Geometry check sheet. Reference: the model listing, model coordinates, mm. A direction names the side the tool comes from. Coordinates: 2 decimals unless noted, no trailing zeros. Loops run counter-clockwise (first coordinate to the right, second up) from the corner with the lowest first, then second, coordinate; pieces in that order, holes last. Notation, with made-up numbers: (-37, 65.5) -> (16, 65.5) arc R14 cw to (16, 87.5) -> close; hole circle Ø8 at (-17, 50). An arc over 180 degrees is marked (long way). Answer as a JSON object with one key per item and string values.
Autodesk Inventor part; units mm, degrees
ref_plane "YZ Plane" through (0, 0, 0) normal (1, 0, 0) x (0, 1, 0)
ref_plane "XZ Plane" through (0, 0, 0) normal (0, 1, 0) x (-1, 0, 0)
ref_plane "XY Plane" through (0, 0, 0) normal (0, 0, 1) x (1, 0, 0)
sketch "Sketch1" plane through (0, 0, 0) normal (0, 1, 0) x (-1, 0, 0)
  line L0 (-25.25, 42.75) -> (25.25, 42.75)
  line L1 (28.25, 39.75) -> (28.25, -40.75)
  line L2 (26.25, -42.75) -> (-25.25, -42.75)
  line L3 (-28.25, -39.75) -> (-28.25, 39.75)
  line L4 (-28.25, 42.75) -> (28.25, -42.75) construction
  line L5 (28.25, 42.75) -> (-28.25, -42.75) construction
  arc A0 (26.25, -42.75) -> (28.25, -40.75) centre (26.25, -40.75) ccw
  arc A1 (-28.25, -39.75) -> (-25.25, -42.75) centre (-25.25, -39.75) ccw
  arc A2 (-25.25, 42.75) -> (-28.25, 39.75) centre (-25.25, 39.75) ccw
  arc A3 (28.25, 39.75) -> (25.25, 42.75) centre (25.25, 39.75) ccw
  line L6 (30.25, -40.75) -> (30.25, 39.75)
  arc A4 (30.25, 39.75) -> (25.25, 44.75) centre (25.25, 39.75) ccw
  line L7 (25.25, 44.75) -> (-25.25, 44.75)
  arc A5 (-25.25, 44.75) -> (-30.25, 39.75) centre (-25.25, 39.75) ccw
  line L8 (-30.25, 39.75) -> (-30.25, -39.75)
  arc A6 (-30.25, -39.75) -> (-25.25, -44.75) centre (-25.25, -39.75) ccw
  line L9 (-25.25, -44.75) -> (26.25, -44.75)
  arc A7 (26.25, -44.75) -> (30.25, -40.75) centre (26.25, -40.75) ccw
  point P0 (0, 0)
  dimension "d0" = 56.5
  dimension "d1" = 85.5
  dimension "d2" = 2
  dimension "d3" = 3
  dimension "d4" = 2
extrude "Extrusion1" add sketch "Sketch1" along normal blind 3
sketch "Sketch2" plane through (0, 0, 0) normal (0, -1, 0) x (1, 0, 0)
  arc A0 (-25.25, 44.75) -> (-30.25, 39.75) centre (-25.25, 39.75) ccw
  line L0 (-25.25, 44.75) -> (25.25, 44.75)
  arc A1 (30.25, 39.75) -> (25.25, 44.75) centre (25.25, 39.75) ccw
  line L1 (30.25, 39.75) -> (30.25, -39.75)
  arc A2 (25.25, -44.75) -> (30.25, -39.75) centre (25.25, -39.75) ccw
  line L2 (25.25, -44.75) -> (-26.25, -44.75)
  arc A3 (-30.25, -40.75) -> (-26.25, -44.75) centre (-26.25, -40.75) ccw
  line L3 (-30.25, -40.75) -> (-30.25, 39.75)
  line L4 (-26.25, -44.75) -> (25.25, -44.75)
  line L5 (30.25, -39.75) -> (30.25, 39.75)
  line L6 (25.25, 44.75) -> (-25.25, 44.75)
  line L7 (-30.25, 39.75) -> (-30.25, -40.75)
  line L8 (-30, -44.5) -> (30, 44.5) construction
  line L9 (30, -44.5) -> (-30, 44.5) construction
  arc A4 (-25.25, 44.75) -> (-30.25, 39.75) centre (-25.25, 39.75) ccw
  arc A5 (30.25, 39.75) -> (25.25, 44.75) centre (25.25, 39.75) ccw
  arc A6 (25.25, -42.75) -> (28.25, -39.75) centre (25.25, -39.75) ccw
  arc A7 (25.25, -44.75) -> (30.25, -39.75) centre (25.25, -39.75) ccw
  arc A8 (-30.25, -40.75) -> (-26.25, -44.75) centre (-26.25, -40.75) ccw
  line L10 (25.25, 40.75) -> (-25.25, 40.75)
  arc A9 (-25.25, 40.75) -> (-26.25, 39.75) centre (-25.25, 39.75) ccw
  line L11 (-26.25, 39.75) -> (-26.25, -40.75)
  line L12 (-26.25, -40.75) -> (25.25, -40.75)
  arc A10 (25.25, -40.75) -> (26.25, -39.75) centre (25.25, -39.75) ccw
  line L13 (26.25, -39.75) -> (26.25, 39.75)
  arc A11 (26.25, 39.75) -> (25.25, 40.75) centre (25.25, 39.75) ccw
  point P0 (0, 0)
  point P1 (-26.25, -40.75)
  dimension "d12" = 4
extrude "Extrusion2" add sketch "Sketch2" along normal blind 2.5
sketch "Sketch3" plane through (25.25, 3, -44.75) normal (0, 0, -1) x (-1, 0, 0)
  line L0 (51.5, -5.5) -> (51.5, 0)
  line L1 (51.5, 0) -> (0, 0)
  line L2 (0, 0) -> (0, 1.5)
  line L3 (0, 1.5) -> (51.5, 1.5)
  line L4 (51.5, 1.5) -> (51.5, 0)
  point P0 (25.25, -3)
  dimension "d9" = 1.5
extrude "Extrusion3" add sketch "Sketch3" against normal blind 2
sketch "Sketch4" plane through (0, -2.5, 0) normal (0, -1, 0) x (1, 0, 0)
  line L0 (25.25, 44.75) -> (-25.25, 44.75)
  line L1 (-30.25, 39.75) -> (-30.25, -40.75)
  line L2 (-26.25, -44.75) -> (25.25, -44.75)
  line L3 (30.25, -39.75) -> (30.25, 39.75)
  line L4 (30, 44.5) -> (-30, -44.5) construction
  line L5 (-30, 44.5) -> (30, -44.5) construction
  line L6 (-26.25, -44.75) -> (25.25, -44.75)
  line L7 (-30.25, 39.75) -> (-30.25, -40.75)
  arc A0 (25.25, -44.75) -> (30.25, -39.75) centre (25.25, -39.75) ccw
  arc A1 (-30.25, -40.75) -> (-26.25, -44.75) centre (-26.25, -40.75) ccw
  arc A2 (-25.25, 44.75) -> (-30.25, 39.75) centre (-25.25, 39.75) ccw
  arc A3 (30.25, 39.75) -> (25.25, 44.75) centre (25.25, 39.75) ccw
  arc A4 (25.25, -44.75) -> (30.25, -39.75) centre (25.25, -39.75) ccw
  line L8 (25.25, -40.75) -> (-26.25, -40.75)
  arc A5 (-30.25, -40.75) -> (-26.25, -44.75) centre (-26.25, -40.75) ccw
  arc A6 (-25.25, 44.75) -> (-30.25, 39.75) centre (-25.25, 39.75) ccw
  arc A7 (30.25, 39.75) -> (25.25, 44.75) centre (25.25, 39.75) ccw
  line L9 (25.25, 44.75) -> (-25.25, 44.75)
  point P0 (0, 0)
  point P1 (-30.25, 39.75)
  point P2 (-30.25, -40.75)
  point P3 (25.25, -44.75)
extrude "Extrusion4" add sketch "Sketch4" along normal blind 2.5
sketch "Sketch5" plane through (25.25, 4.5, -44.75) normal (0, 0, -1) x (-1, 0, 0)
  line L0 (51.5, -9.5) -> (0, -9.5)
  line L1 (18.25, -9.5) -> (32.25, -9.5)
  line L2 (32.25, -9.5) -> (32.25, -4.5)
  line L3 (32.25, -4.5) -> (18.25, -4.5)
  line L4 (18.25, -4.5) -> (18.25, -9.5)
  line L5 (18.25, -9.5) -> (32.25, -4.5) construction
  line L6 (32.25, -9.5) -> (18.25, -4.5) construction
  point P0 (25.25, -4.5)
  point P1 (25.25, -7)
  dimension "d16" = 14
  dimension "d17" = 0
  dimension "d18" = 5
extrude "Extrusion5" cut sketch "Sketch5" against normal blind 10
sketch "Sketch6" plane through (-30.25, 3, -40.75) normal (-1, 0, 0) x (0, 0, 1)
  line L0 (1, 0) -> (80.5, 0)
  line L1 (4.6696, 0) -> (13.8622, 0)
  line L2 (13.8622, 0) -> (13.8622, -2)
  line L3 (13.8622, -2) -> (4.6696, -2)
  line L4 (4.6696, -2) -> (4.6696, 0)
  line L5 (20.7687, 0) -> (27.5371, 0)
  line L6 (27.5371, 0) -> (27.5371, -2)
  line L7 (27.5371, -2) -> (20.7687, -2)
  line L8 (20.7687, -2) -> (20.7687, 0)
  line L9 (34.3481, 0) -> (41.1165, 0)
  line L10 (41.1165, 0) -> (41.1165, -2)
  line L11 (41.1165, -2) -> (34.3481, -2)
  line L12 (34.3481, -2) -> (34.3481, 0)
  arc A0 (49.8136, 0) -> (55.8136, 0) centre (52.8136, 1.25) ccw
  line L13 (-2, 1.5) -> (-2, 0)
  line L14 (80.5, -8) -> (0, -8)
  line L15 (49.8136, 0) -> (55.8136, 0)
  point P0 (40.75, -3)
  dimension "d21" = 6.6696
  dimension "d22" = 9.1926
  dimension "d23" = 22.7687
  dimension "d25" = 6.7684
  dimension "d26" = 6.7684
  dimension "d27" = 36.3481
  dimension "d28" = 51.8136
  dimension "d29" = 6
  dimension "d30" = 2
extrude "Extrusion6" cut sketch "Sketch6" against normal up to surface (2 mm away)
sketch "Sketch7" plane through (-25.25, 3, 44.75) normal (0, 0, 1) x (1, 0, 0)
  line L0 (50.5, 0) -> (0, 0)
  line L1 (-0.7188, 0) -> (12.8798, 0)
  line L2 (12.8798, 0) -> (12.8798, -2)
  line L3 (12.8798, -2) -> (-0.7188, -2)
  line L4 (-0.7188, -2) -> (-0.7188, 0)
  line L5 (17.4418, 0) -> (31.0404, 0)
  line L6 (31.0404, 0) -> (31.0404, -2)
  line L7 (31.0404, -2) -> (17.4418, -2)
  line L8 (17.4418, -2) -> (17.4418, 0)
  line L9 (34.977, 0) -> (51.34, 0)
  line L10 (51.34, 0) -> (51.34, -2)
  line L11 (51.34, -2) -> (34.977, -2)
  line L12 (34.977, -2) -> (34.977, 0)
  line L13 (-3, -3) -> (-3, 0)
  point P0 (25.25, -3)
  dimension "d33" = 2
  dimension "d34" = 2.2812
  dimension "d35" = 13.5986
  dimension "d36" = 20.4418
  dimension "d37" = 13.5986
  dimension "d38" = 37.977
  dimension "d39" = 16.363
extrude "Extrusion7" cut sketch "Sketch7" against normal blind 5
properties part number "piholder-v2"
1. Section check A-A, the plane x = -3. Record the boundary of the cut face in (y, z), then the cut area to 3 significant figures.
Evaluation:
{"outline": "(-5, -34.75) -> (-2.5, -34.75) -> (-2.5, 40.75) -> (0, 40.75) -> (0, 42.75) -> (1, 42.75) -> (1, 44.75) -> (-5, 44.75) -> close; (0, -44.75) -> (4.5, -44.75) -> (4.5, -42.75) -> (0, -42.75) -> close", "area": "220 mm^2"}
2. Thickness scan on probe 1 along X at (y, z) = (2.25, -25); probe 2 along Z at (x, y) = (25.5, 0.25); probe 3 along X at (y, z) = (-1.25, 28). Record the ranges inside material, lowest first. Write a range as from..to.
Evaluation:
{"probe 1": "x = -30.25..-28.25, 28.25..30.25", "probe 2": "z = -44.74..-42.74, 42.74..44.74", "probe 3": "x = -30.25..-26.25, 26.25..30.25"}
3. Section check B-B, the plane z = 26. Record the boundary of the cut face in (x, y), then the cut area to 3 significant figures.
Evaluation:
{"outline": "(-30.25, -5) -> (30.25, -5) -> (30.25, 3) -> (28.25, 3) -> (28.25, 0) -> (26.25, 0) -> (26.25, -2.5) -> (-26.25, -2.5) -> (-26.25, 0) -> (-28.25, 0) -> (-28.25, 3) -> (-30.25, 3) -> close", "area": "183 mm^2"}
4. Depth check by flat-ended pin: P1, Ø1.6, axis at y = 1.5, z = 43.5, coming from the +X side; P2, Ø1, axis at x = -29, y = 2, coming from the -Z side; P3, Ø8, axis at x = 19, z = -33, coming from the +Y side. Enter the tip coordinate at first touch or a pass-through.
Evaluation:
{"P1": "stops at x = 29.29", "P2": "stops at z = -44.06", "P3": "stops at y = -2.5"}
5. Section check C-C, the plane x = 18. Record the boundary of the cut face in (y, z), then the cut area to 3 significant figures.
Evaluation:
{"outline": "(-5, -44.75) -> (4.5, -44.75) -> (4.5, -42.75) -> (0, -42.75) -> (0, -40.75) -> (-2.5, -40.75) -> (-2.5, 40.75) -> (0, 40.75) -> (0, 42.75) -> (1, 42.75) -> (1, 44.75) -> (-5, 44.75) -> close", "area": "255 mm^2"}
6. Mould release check, pull along Z, two halves, no side actions. Record for faces 6 (the face through (-29, 2, -19.981)), 7 (the face through (-30.25, -1, 0)), 8 (the face through (27.73, 1.48, 41.44)), 9 (the face through (-1, 1, -44.75)): released by +Z, released by -Z, zero draft, split by the parting line, or undercut.
Evaluation:
{"face 6": "undercut", "face 7": "zero draft", "face 8": "undercut", "face 9": "released by -Z"}
7. Tool access check on faces 1 (the face through (7, -3, -41)), 2 (the face through (-27.68, 1.48, -42.15)), 3 (the face through (18, 1, 44)), 4 (the face through (-29, 2, 0.366)), 5 (the face through (0, -4, -34.75)). Record the directions out of +Z, -Z, +X, -X, +Y, -Y that give a thin tool (end or side, any length) a straight path to the whole face; none if there is none.
Evaluation:
{"face 1": "-Z, -Y", "face 2": "+Y", "face 3": "+Z, +Y", "face 4": "-X, +Y", "face 5": "-Z, +Y, -Y"}
